Could you check a few things on this model? Use its own coordinates, in mm. Coordinates: 2 decimals unless noted, no trailing zeros. Loops run counter-clockwise (first coordinate to the right, second up) from the corner with the lowest first, then second, coordinate; pieces in that order, holes last.
from build123d import *

# Parameters (mm, degrees)
SKETCH1_R           = 19.05
BOSS_EXTRUDE1_DEPTH = 4.7625


# Read off the part's stored shape, not the designer's step: Imported1
with BuildPart() as part:
    # Sketch1 → Boss-Extrude1 (new body)
    with BuildSketch(Plane.XY.offset(2.38125)):
        with Locations(Location((0, 0, 0), (0, 0, 180))):
            Circle(SKETCH1_R)
        with BuildLine():
            Line((1.908812995, 11.759820716), (1.810138608, 13.497531825))
            ThreePointArc((1.810138608, 13.497531825), (1.334833561, 13.552792572), (0.857880531, 13.591321069))
            Line((0.857880531, 13.591321069), (0.422091522, 11.90625))
            Line((0.422091522, 11.90625), (-0.422091522, 11.90625))
            Line((-0.422091522, 11.90625), (-0.857880531, 13.591321069))
            ThreePointArc((-0.857880531, 13.591321069), (-1.334833561, 13.552792582), (-1.810138607, 13.497531835))
            Line((-1.810138607, 13.497531835), (-1.908812995, 11.759820716))
            Line((-1.908812995, 11.759820716), (-2.736775298, 11.595128774))
            Line((-2.736775298, 11.595128774), (-3.492931801, 13.162803457))
            ThreePointArc((-3.492931801, 13.162803457), (-3.953203777, 13.031966364), (-4.408595133, 12.885040022))
            Line((-4.408595133, 12.885040022), (-4.166362899, 11.161468116))
            Line((-4.166362899, 11.161468116), (-4.946286334, 10.838413252))
            Line((-4.946286334, 10.838413252), (-5.993751661, 12.228446689))
            ThreePointArc((-5.993751661, 12.228446689), (-6.41965459, 12.010328986), (-6.837631821, 11.777383347))
            Line((-6.837631821, 11.777383347), (-6.263801813, 10.134186556))
            Line((-6.263801813, 10.134186556), (-6.965714361, 9.665183587))
            Line((-6.965714361, 9.665183587), (-8.264235006, 10.824157574))
            ThreePointArc((-8.264235006, 10.824157574), (-8.639401676, 10.527141401), (-9.003902152, 10.217128434))
            Line((-9.003902152, 10.217128434), (-8.120526336, 8.717453891))
            Line((-8.120526336, 8.717453891), (-8.717453891, 8.120526336))
            Line((-8.717453891, 8.120526336), (-10.217128434, 9.003902152))
            ThreePointArc((-10.217128434, 9.003902152), (-10.527141401, 8.639401676), (-10.824157574, 8.264235006))
            Line((-10.824157574, 8.264235006), (-9.665183587, 6.965714361))
            Line((-9.665183587, 6.965714361), (-10.134186556, 6.263801813))
            Line((-10.134186556, 6.263801813), (-11.777383347, 6.837631821))
            ThreePointArc((-11.777383347, 6.837631821), (-12.010328986, 6.41965459), (-12.228446689, 5.993751661))
            Line((-12.228446689, 5.993751661), (-10.838413252, 4.946286334))
            Line((-10.838413252, 4.946286334), (-11.161468116, 4.166362899))
            Line((-11.161468116, 4.166362899), (-12.885040022, 4.408595133))
            ThreePointArc((-12.885040022, 4.408595133), (-13.031966364, 3.953203777), (-13.162803457, 3.492931801))
            Line((-13.162803457, 3.492931801), (-11.595128774, 2.736775298))
            Line((-11.595128774, 2.736775298), (-11.759820716, 1.908812995))
            Line((-11.759820716, 1.908812995), (-13.497531835, 1.810138607))
            ThreePointArc((-13.497531835, 1.810138607), (-13.552792582, 1.334833561), (-13.591321069, 0.857880531))
            Line((-13.591321069, 0.857880531), (-11.90625, 0.422091522))
            Line((-11.90625, 0.422091522), (-11.90625, -0.422091522))
            Line((-11.90625, -0.422091522), (-13.591321069, -0.857880531))
            ThreePointArc((-13.591321069, -0.857880531), (-13.552792582, -1.334833561), (-13.497531835, -1.810138607))
            Line((-13.497531835, -1.810138607), (-11.759820716, -1.908812995))
            Line((-11.759820716, -1.908812995), (-11.595128774, -2.736775298))
            Line((-11.595128774, -2.736775298), (-13.162803457, -3.492931801))
            ThreePointArc((-13.162803457, -3.492931801), (-13.031966364, -3.953203777), (-12.885040022, -4.408595133))
            Line((-12.885040022, -4.408595133), (-11.161468116, -4.166362899))
            Line((-11.161468116, -4.166362899), (-10.838413252, -4.946286334))
            Line((-10.838413252, -4.946286334), (-12.228446689, -5.993751661))
            ThreePointArc((-12.228446689, -5.993751661), (-12.010328986, -6.41965459), (-11.777383347, -6.837631821))
            Line((-11.777383347, -6.837631821), (-10.134186556, -6.263801813))
            Line((-10.134186556, -6.263801813), (-9.665183587, -6.965714361))
            Line((-9.665183587, -6.965714361), (-10.824157574, -8.264235006))
            ThreePointArc((-10.824157574, -8.264235006), (-10.527141401, -8.639401676), (-10.217128434, -9.003902152))
            Line((-10.217128434, -9.003902152), (-8.717453891, -8.120526336))
            Line((-8.717453891, -8.120526336), (-8.120526336, -8.717453891))
            Line((-8.120526336, -8.717453891), (-9.003902152, -10.217128434))
            ThreePointArc((-9.003902152, -10.217128434), (-8.639401676, -10.527141401), (-8.264235006, -10.824157574))
            Line((-8.264235006, -10.824157574), (-6.965714361, -9.665183587))
            Line((-6.965714361, -9.665183587), (-6.263801813, -10.134186556))
            Line((-6.263801813, -10.134186556), (-6.837631821, -11.777383347))
            ThreePointArc((-6.837631821, -11.777383347), (-6.41965459, -12.010328986), (-5.993751661, -12.228446689))
            Line((-5.993751661, -12.228446689), (-4.946286334, -10.838413252))
            Line((-4.946286334, -10.838413252), (-4.166362899, -11.161468116))
            Line((-4.166362899, -11.161468116), (-4.408595133, -12.885040022))
            ThreePointArc((-4.408595133, -12.885040022), (-3.953203777, -13.031966364), (-3.492931801, -13.162803457))
            Line((-3.492931801, -13.162803457), (-2.736775298, -11.595128774))
            Line((-2.736775298, -11.595128774), (-1.908812995, -11.759820716))
            Line((-1.908812995, -11.759820716), (-1.810138607, -13.497531835))
            ThreePointArc((-1.810138607, -13.497531835), (-1.334833561, -13.552792582), (-0.857880531, -13.591321069))
            Line((-0.857880531, -13.591321069), (-0.422091522, -11.90625))
            Line((-0.422091522, -11.90625), (0.422091522, -11.90625))
            Line((0.422091522, -11.90625), (0.857880531, -13.591321069))
            ThreePointArc((0.857880531, -13.591321069), (1.334833561, -13.552792582), (1.810138607, -13.497531835))
            Line((1.810138607, -13.497531835), (1.908812995, -11.759820716))
            Line((1.908812995, -11.759820716), (2.736775298, -11.595128774))
            Line((2.736775298, -11.595128774), (3.492931801, -13.162803457))
            ThreePointArc((3.492931801, -13.162803457), (3.953203777, -13.031966364), (4.408595133, -12.885040022))
            Line((4.408595133, -12.885040022), (4.166362899, -11.161468116))
            Line((4.166362899, -11.161468116), (4.946286334, -10.838413252))
            Line((4.946286334, -10.838413252), (5.993751661, -12.228446689))
            ThreePointArc((5.993751661, -12.228446689), (6.41965459, -12.010328986), (6.837631821, -11.777383347))
            Line((6.837631821, -11.777383347), (6.263801813, -10.134186556))
            Line((6.263801813, -10.134186556), (6.965714361, -9.665183587))
            Line((6.965714361, -9.665183587), (8.264235006, -10.824157574))
            ThreePointArc((8.264235006, -10.824157574), (8.639401676, -10.527141401), (9.003902152, -10.217128434))
            Line((9.003902152, -10.217128434), (8.120526336, -8.717453891))
            Line((8.120526336, -8.717453891), (8.717453891, -8.120526336))
            Line((8.717453891, -8.120526336), (10.217128434, -9.003902152))
            ThreePointArc((10.217128434, -9.003902152), (10.527141401, -8.639401676), (10.824157574, -8.264235006))
            Line((10.824157574, -8.264235006), (9.665183587, -6.965714361))
            Line((9.665183587, -6.965714361), (10.134186556, -6.263801813))
            Line((10.134186556, -6.263801813), (11.777383347, -6.837631821))
            ThreePointArc((11.777383347, -6.837631821), (12.010328986, -6.41965459), (12.228446689, -5.993751661))
            Line((12.228446689, -5.993751661), (10.838413252, -4.946286334))
            Line((10.838413252, -4.946286334), (11.161468116, -4.166362899))
            Line((11.161468116, -4.166362899), (12.885040022, -4.408595133))
            ThreePointArc((12.885040022, -4.408595133), (13.031966364, -3.953203777), (13.162803457, -3.492931801))
            Line((13.162803457, -3.492931801), (11.595128774, -2.736775298))
            Line((11.595128774, -2.736775298), (11.759820716, -1.908812995))
            Line((11.759820716, -1.908812995), (13.497531835, -1.810138607))
            ThreePointArc((13.497531835, -1.810138607), (13.552792582, -1.334833561), (13.591321069, -0.857880531))
            Line((13.591321069, -0.857880531), (11.90625, -0.422091522))
            Line((11.90625, -0.422091522), (11.90625, 0.422091522))
            Line((11.90625, 0.422091522), (13.591321069, 0.857880531))
            ThreePointArc((13.591321069, 0.857880531), (13.552792582, 1.334833561), (13.497531835, 1.810138607))
            Line((13.497531835, 1.810138607), (11.759820716, 1.908812995))
            Line((11.759820716, 1.908812995), (11.595128774, 2.736775298))
            Line((11.595128774, 2.736775298), (13.162803457, 3.492931801))
            ThreePointArc((13.162803457, 3.492931801), (13.031966364, 3.953203777), (12.885040022, 4.408595133))
            Line((12.885040022, 4.408595133), (11.161468116, 4.166362899))
            Line((11.161468116, 4.166362899), (10.838413252, 4.946286334))
            Line((10.838413252, 4.946286334), (12.228446689, 5.993751661))
            ThreePointArc((12.228446689, 5.993751661), (12.010328986, 6.41965459), (11.777383347, 6.837631821))
            Line((11.777383347, 6.837631821), (10.134186556, 6.263801813))
            Line((10.134186556, 6.263801813), (9.665183587, 6.965714361))
            Line((9.665183587, 6.965714361), (10.824157574, 8.264235006))
            ThreePointArc((10.824157574, 8.264235006), (10.527141401, 8.639401676), (10.217128434, 9.003902152))
            Line((10.217128434, 9.003902152), (8.717453891, 8.120526336))
            Line((8.717453891, 8.120526336), (8.120526336, 8.717453891))
            Line((8.120526336, 8.717453891), (9.003902152, 10.217128434))
            ThreePointArc((9.003902152, 10.217128434), (8.639401676, 10.527141401), (8.264235006, 10.824157574))
            Line((8.264235006, 10.824157574), (6.965714361, 9.665183587))
            Line((6.965714361, 9.665183587), (6.263801813, 10.134186556))
            Line((6.263801813, 10.134186556), (6.837631821, 11.777383347))
            ThreePointArc((6.837631821, 11.777383347), (6.41965459, 12.010328986), (5.993751661, 12.228446689))
            Line((5.993751661, 12.228446689), (4.946286334, 10.838413252))
            Line((4.946286334, 10.838413252), (4.166362899, 11.161468116))
            Line((4.166362899, 11.161468116), (4.408595133, 12.885040022))
            ThreePointArc((4.408595133, 12.885040022), (3.953203777, 13.031966364), (3.492931801, 13.162803457))
            Line((3.492931801, 13.162803457), (2.736775298, 11.595128774))
            Line((2.736775298, 11.595128774), (1.908812995, 11.759820716))
        make_face(mode=Mode.SUBTRACT)
    extrude(amount=-BOSS_EXTRUDE1_DEPTH)


solid = part.part
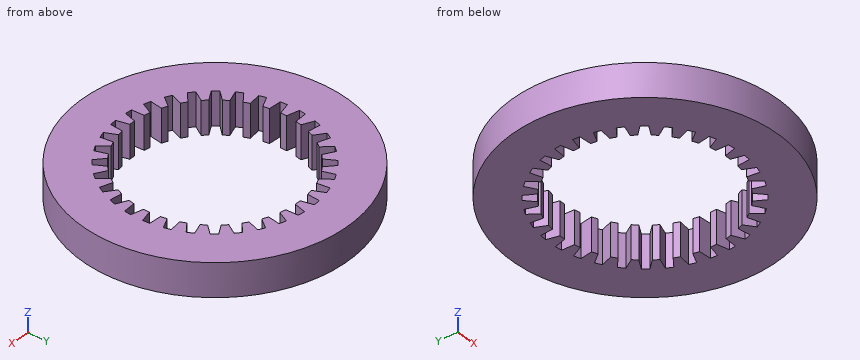
1) Imagine slicing it at A-A on x = -14.5. List the corners of the cut face in (y, z) for me.
2) Will these pins go through, and if not, where does the flat tip stop? pin 1 (1.5 mm diameter, centred on y = 14.5, z = 0.5, fed in from +X); pin 2 (0.7 mm diameter, centred on x = 0, z = 1, fed in from -Y); pin 3 (0.7 mm diameter, centred on x = 0, z = 0.5, fed in from +Y).
3) If I drill on L1, parallel to Y at x = -8.5, z = 1.3; L2, parallel to X at y = 11.5, z = -0.95; L3, parallel to Y at x = -11, z = 0.4, over which ranges is the centre line in solid material (lowest first)?
Solved:
1. outline: (-12.36, -2.38) - (12.36, -2.38) - (12.36, 2.38) - (-12.36, 2.38) - close
2. pin 1: stops at x = 13.18
2. pin 2: stops at y = -19.05
2. pin 3: stops at y = 19.05
3. L1: y = -17.05 to -10.64, -9.36 to -8.34, 8.34 to 9.36, 10.64 to 17.05
3. L2: x = -15.19 to -6.74, -5.44 to -4.21, 4.21 to 5.44, 6.74 to 15.19
3. L3: y = -15.55 to -6.57, -5.07 to -4.56, 4.56 to 5.07, 6.57 to 15.55
